Verification items for the finished model (mm, model axes). Face numbers are marked on the shaded views. A direction names the side the tool comes from. Give positions to 0.01 mm unless a question says otherwise; leave off trailing zeros. Loops run counter-clockwise (first coordinate to the right, second up) from the corner with the lowest first, then second, coordinate; pieces in that order, holes last. Notation, with made-up numbers: M -13.75,28.5 L 18.25,28.5 A22 ccw 18.25,35.5 Z; hole C -15.5,40 d5. An arc over 180 degrees is marked long. Use a Markdown table: item, result.
Autodesk Inventor part; units mm, degrees
ref_plane "YZ Plane" through (0, 0, 0) normal (1, 0, 0) x (0, 1, 0)
ref_plane "XZ Plane" through (0, 0, 0) normal (0, 1, 0) x (-1, 0, 0)
ref_plane "XY Plane" through (0, 0, 0) normal (0, 0, 1) x (1, 0, 0)
sketch "Sketch1" plane through (0, 0, 0) normal (0, 0, 1) x (1, 0, 0)
  line L0 (-13.75, -10.5) -> (13.75, -10.5)
  line L1 (13.75, -10.5) -> (13.75, 10.5)
  line L2 (13.75, 10.5) -> (-13.75, 10.5)
  line L3 (-13.75, 10.5) -> (-13.75, -10.5)
  line L4 (-13.75, -10.5) -> (13.75, 10.5) construction
  line L5 (13.75, -10.5) -> (-13.75, 10.5) construction
  line L6 (-8.5, 8.5) -> (8.5, 8.5)
  line L7 (8.5, 8.5) -> (8.5, 3.5)
  line L8 (8.5, 3.5) -> (-8.5, 3.5)
  line L9 (-8.5, 3.5) -> (-8.5, 8.5)
  line L10 (-8.5, 8.5) -> (8.5, 3.5) construction
  line L11 (8.5, 8.5) -> (-8.5, 3.5) construction
  line L12 (-19.25, 0) -> (19.25, 0) construction
  line L13 (-8.5, -8.5) -> (8.5, -8.5)
  line L14 (8.5, -8.5) -> (8.5, -3.5)
  line L15 (8.5, -3.5) -> (-8.5, -3.5)
  line L16 (-8.5, -3.5) -> (-8.5, -8.5)
  line L17 (0, -14.7) -> (0, 14.7) construction
  circle A0 centre (0, 0) radius 1.5
  point P0 (0, 6)
  point P1 (8.5, 6)
  point P2 (11.5, -8.1)
  point P3 (11.5, -6.3)
  point P4 (11.5, -4.5)
  point P5 (11.5, -0.9)
  point P6 (11.5, -2.7)
  point P7 (11.5, 8.1)
  point P8 (11.5, 6.3)
  point P9 (11.5, 4.5)
  point P10 (11.5, 0.9)
  point P11 (11.5, 2.7)
  point P12 (-11.5, -8.1)
  point P13 (-11.5, -6.3)
  point P14 (-11.5, -4.5)
  point P15 (-11.5, -0.9)
  point P16 (-11.5, -2.7)
  point P17 (-11.5, 8.1)
  point P18 (-11.5, 6.3)
  point P19 (-11.5, 4.5)
  point P20 (-11.5, 2.7)
  point P21 (-11.5, 0.9)
  dimension "d0" = 21
  dimension "d1" = 27.5
  dimension "d28" = 17
  dimension "d29" = 5
  dimension "d30" = 2
  dimension "d31" = 1.8
  dimension "d32" = 1.8
  dimension "d33" = 1.8
  dimension "d34" = 1.8
  dimension "d35" = 0.9
  dimension "d36" = 2.25
  dimension "d44" = 3
extrude "Extrusion1" add sketch "Sketch1" against normal blind 1 contours L3 L2 L1 L0 | A0
hole "Hole2" at (11.5, -8.1, 0) at (11.5, -6.3, 0) at (11.5, -4.5, 0) at (11.5, -0.9, 0) at (11.5, -2.7, 0) at (11.5, 8.1, 0) at (11.5, 6.3, 0) at (11.5, 4.5, 0) at (11.5, 2.7, 0) at (11.5, 0.9, 0) at (-11.5, 8.1, 0) at (-11.5, 6.3, 0) at (-11.5, 4.5, 0) at (-11.5, 2.7, 0) at (-11.5, 0.9, 0) at (-11.5, -0.9, 0) at (-11.5, -2.7, 0) at (-11.5, -4.5, 0) at (-11.5, -6.3, 0) at (-11.5, -8.1, 0) direction (0, 0, -1) diameter 0.5 end through all
extrude "Extrusion3" add sketch "Sketch1" along normal blind 9.5 contours A0
thread "Thread3"
fillet "Fillet3" radius 1 1 edges at (-1.5, 0, 0)
properties part number "Soporte"
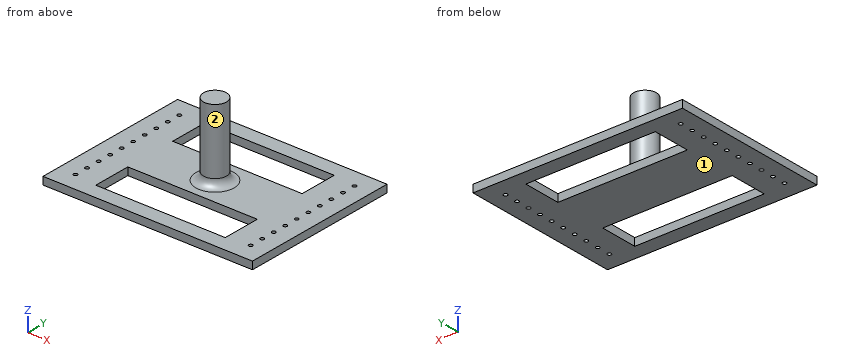
(1) Cross-section at D-D on z = 2.75. Record the cut outline in (x, y), then the cut area to 3 significant figures.
Results below:
| item | result |
|---|---|
| outline | C 0,0 d3 |
| area | 7.07 mm^2 |
(2) Cross-section at A-A on z = -0.5. State how many separate pieces and enclosed holes the cut face has, then the cut area to 3 significant figures.
Results below:
| item | result |
|---|---|
| separate pieces | 1 |
| enclosed holes | 22 |
| area | 404 mm^2 |
(3) Gauge pin test, flat end, axial feed: P1, Ø1.5, axis at x = -0.5, y = 6.5, coming from the +Z side. Record the tip position at first contact, or that the pin passes through.
Results below:
| item | result |
|---|---|
| P1 | through |
(4) Cross-section at C-C on y = 0. Record the cut outline in (x, z), then the cut area to 3 significant figures.
Results below:
| item | result |
|---|---|
| outline | M -13.75,-1 L 13.75,-1 L 13.75,0 L 2.5,0 A1 cw 1.5,1 L 1.5,9.5 L -1.5,9.5 L -1.5,1 A1 cw -2.5,0 L -13.75,0 Z |
| area | 56.4 mm^2 |
(5) Cross-section at B-B on x = -7. Record the cut outline in (y, z).
Results below:
| item | result |
|---|---|
| outline | M -10.5,-1 L -8.5,-1 L -8.5,0 L -10.5,0 Z; M -3.5,-1 L 3.5,-1 L 3.5,0 L -3.5,0 Z; M 8.5,-1 L 10.5,-1 L 10.5,0 L 8.5,0 Z |
(6) Material ranges on line 1 (X direction, y = 0.9, z = -0.45); line 2 (X direction, y = -8.1, z = -0.3); line 3 (Z direction, x = 10.5, y = -0.25), recorded low to high.
Results below:
| item | result |
|---|---|
| line 1 | -13.75 to -11.75, -11.25 to 11.25, 11.75 to 13.75 |
| line 2 | -13.75 to -11.75, -11.25 to -8.5, 8.5 to 11.25, 11.75 to 13.75 |
| line 3 | -1 to 0 |
(7) Set-up check for the marked faces 1 and 2: record each of +Z, -Z, +X, -X, +Y, -Y from which the full face is reachable in a straight line by a thin tool's end or side.
Results below:
| item | result |
|---|---|
| face 1 | -Z, +X, -X, +Y, -Y |
| face 2 | +Z |
